from build123d import *

# Parameters (mm, degrees)
CYLINDER980_R     = 1
CYLINDER980_DEPTH = 20
CYLINDER977_R     = 1
CYLINDER977_DEPTH = 20
CYLINDER976_R     = 1
CYLINDER976_DEPTH = 20
CYLINDER979_R     = 1
CYLINDER979_DEPTH = 20
TUBE089_R         = 9
TUBE089_R_2       = 2.55
TUBE089_DEPTH     = 10


with BuildPart() as obj1:
    # Cylinder980 → Cylinder980 (new body)
    with BuildSketch(Plane(origin=(4.5, -4.5, -88), x_dir=(0, 1, 0), z_dir=(0, 0, 1))):
        Circle(CYLINDER980_R)
    extrude(amount=CYLINDER980_DEPTH)


with BuildPart() as obj2:
    # Cylinder977 → Cylinder977 (new body)
    with BuildSketch(Plane(origin=(4.5, 4.5, -88), x_dir=(-1, 0, 0), z_dir=(0, 0, 1))):
        Circle(CYLINDER977_R)
    extrude(amount=CYLINDER977_DEPTH)


with BuildPart() as obj3:
    # Cylinder976 → Cylinder976 (new body)
    with BuildSketch(Plane(origin=(-4.5, 4.5, -88), x_dir=(0, -1, 0), z_dir=(0, 0, 1))):
        Circle(CYLINDER976_R)
    extrude(amount=CYLINDER976_DEPTH)


with BuildPart() as compound809:
    # Cylinder979 → Cylinder979 (new body)
    with BuildSketch(Plane(origin=(-4.5, -4.5, -88), x_dir=(1, 0, 0), z_dir=(0, 0, 1))):
        Circle(CYLINDER979_R)
    extrude(amount=CYLINDER979_DEPTH)

    # Compound809: union obj1, obj2, obj3
    add(obj1.part)
    add(obj2.part)
    add(obj3.part)


with BuildPart() as compound809_1:
    # Compound809 placement: moved
    add(compound809.part.moved(Location((0, 0, 91))))


with BuildPart() as cut413:
    # Tube089 → Tube089 (new body)
    with BuildSketch(Plane.XY.offset(19)):
        Circle(TUBE089_R)
        Circle(TUBE089_R_2, mode=Mode.SUBTRACT)
    extrude(amount=TUBE089_DEPTH)

    # Cut413: cut Compound809
    add(compound809_1.part, mode=Mode.SUBTRACT)


solid = cut413.part
Can you work these out from the model? Positions are in its coordinate system, mm. A direction names the side the tool comes from. Give positions to 0.01 mm unless a question says otherwise; leave off trailing zeros. Loops run counter-clockwise (first coordinate to the right, second up) from the corner with the lowest first, then second, coordinate; pieces in that order, holes last. Notation, with made-up numbers: (-10.5, 59.5) - (8.5, 59.5) arc R20 ccw to (8.5, 65.5) - close; hole circle Ø10 at (-5, -21). An arc over 180 degrees is marked (long way). One line per item, written item: value.
(1) I'm going to push flat-ended pins straight in: pin 1 (1 mm diameter, centred on x = 4.5, y = -4.5, fed in from -Z); pin 2 (2 mm diameter, centred on y = -5, z = 20.5, fed in from -X); pin 3 (1.5 mm diameter, centred on y = -6, z = 22, fed in from +X); pin 4 (2 mm diameter, centred on x = -4, y = 5, fed in from -Z). Where does each tip first touch, or does it pass through?
Verdict:
pin 1: z = 23
pin 2: x = -8.06
pin 3: x = 7.31
pin 4: z = 19
(2) If we section it at A-A, the plane x = 0: List the corners of the cut face in (y, z) for me, plus the area to 3 significant figures.
Verdict:
outline: (-9, 19) - (-2.55, 19) - (-2.55, 29) - (-9, 29) - close; (2.55, 19) - (9, 19) - (9, 29) - (2.55, 29) - close
area: 129 mm^2
(3) If we mould it in two halves opening along Y, with no side actions, what happens to faces 1 (the face through (2, -2, 19)), 2 (the face through (-1.172, 8.923, 23.93)), 3 (the face through (-3.51, 4.63, 20.97))? For each: released by +Y, released by -Y, zero draft, split by the parting line, or undercut.
Verdict:
face 1: zero draft
face 2: split by the parting line
face 3: undercut
(4) If we section it at D-D, the plane z = 25.5: List the corners of the cut face in (x, y) for me, plus the area to 3 significant figures.
Verdict:
outline: circle Ø18 at (0, 0); hole circle Ø5.1 at (0, 0)
area: 234 mm^2
(5) If we section it at C-C, the plane z = 21: List the corners of the cut face in (x, y) for me.
Verdict:
outline: circle Ø18 at (0, 0); hole circle Ø2 at (-4.5, -4.5); hole circle Ø2 at (-4.5, 4.5); hole circle Ø5.1 at (0, 0); hole circle Ø2 at (4.5, -4.5); hole circle Ø2 at (4.5, 4.5)
(6) On a 3-axis mill with a long thin cutter (end or side, diameter ignored), from which of +Z, -Z, +X, -X, +Y, -Y can I reach the whole of each face in a straight line? I mean faces 4 (the face through (5, 4, 23)), 5 (the face through (2, -2, 29)). Say none if no direction works.
Verdict:
face 4: -Z
face 5: +Z, +X, -X, +Y, -Y
(7) I need wall thicknesses on line 1 along X through (y, z) = (-4.5, 21.9); line 2 along X through (y, z) = (3.75, 22.25); line 3 along Y through (x, z) = (0, 25.25). Which ranges of each line are inside material? Lowest first, please.
Verdict:
line 1: -7.79 to -5.5, -3.5 to 3.5, 5.5 to 7.79
line 2: -8.18 to -5.16, -3.84 to 3.84, 5.16 to 8.18
line 3: -9 to -2.55, 2.55 to 9
